from build123d import *

# Parameters (mm, degrees)
SKETCH_1_R          = 1.1
SKETCH_1_W          = 26
SKETCH_1_H          = 32.5
EXTRUDE_1_DEPTH     = 11
SKETCH_3_R          = 1.1
EXTRUDE_2_DEPTH     = 2
SKETCH_2_R          = 1.1
CUT_EXTRUDE_1_DEPTH = 50.401315772
SKETCH_4_W          = 8
SKETCH_4_H          = 17
CUT_EXTRUDE_3_DEPTH = 10
SKETCH_5_R          = 2.5
CUT_EXTRUDE_4_DEPTH = 0.4
SKETCH_6_W          = 3.5
SKETCH_6_H          = 13
SKETCH_6_W_2        = 10
SKETCH_6_H_2        = 2
CUT_EXTRUDE_6_DEPTH = 3
FILLET_1_R          = 7.5
SKETCH_7_W          = 3
SKETCH_7_H          = 13
CUT_EXTRUDE_7_DEPTH = 49.449355001


with BuildPart() as part:
    # ｽｹｯﾁ1 → ﾎﾞｽ - 押し出し1 (new body)
    with BuildSketch(Plane.XY):
        with BuildLine():
            Line((26.8, 35.5), (26.8, -3.5))
            ThreePointArc((26.8, -3.5), (26.067766953, -5.267766953), (24.3, -6))
            Line((24.3, -6), (-2.5, -6))
            ThreePointArc((-2.5, -6), (-4.267766953, -5.267766953), (-5, -3.5))
            Line((-5, -3.5), (-5, 33))
            ThreePointArc((-5, 33), (-4.267766953, 34.767766953), (-2.5, 35.5))
            Line((-2.5, 35.5), (26.8, 35.5))
        make_face()
        with Locations((-2.5, 33)):
            Circle(SKETCH_1_R, mode=Mode.SUBTRACT)
        with Locations((-2.5, -3.5)):
            Circle(SKETCH_1_R, mode=Mode.SUBTRACT)
        with Locations((21.8, -3.5)):
            Circle(SKETCH_1_R, mode=Mode.SUBTRACT)
        with Locations((13, 16.25)):
            Rectangle(SKETCH_1_W, SKETCH_1_H, mode=Mode.SUBTRACT)
    extrude(amount=EXTRUDE_1_DEPTH)

    # ｽｹｯﾁ3 → ﾎﾞｽ - 押し出し2 (add)
    with BuildSketch(Plane(origin=(0, 0, 11), x_dir=(-1, 0, 0), z_dir=(0, 0, -1))):
        with BuildLine():
            Line((5, -3.5), (5, 33))
            ThreePointArc((5, 33), (4.267766953, 34.767766953), (2.5, 35.5))
            Line((2.5, 35.5), (-26.8, 35.5))
            Line((-26.8, 35.5), (-26.8, -3.5))
            ThreePointArc((-26.8, -3.5), (-26.067766953, -5.267766953), (-24.3, -6))
            Line((-24.3, -6), (2.5, -6))
            ThreePointArc((2.5, -6), (4.267766953, -5.267766953), (5, -3.5))
        make_face()
        with Locations((-21.8, -3.5)):
            Circle(SKETCH_3_R, mode=Mode.SUBTRACT)
        with Locations((2.5, -3.5)):
            Circle(SKETCH_3_R, mode=Mode.SUBTRACT)
        with Locations((2.5, 33)):
            Circle(SKETCH_3_R, mode=Mode.SUBTRACT)
    extrude(amount=-EXTRUDE_2_DEPTH)

    # ｽｹｯﾁ2 → ｶｯﾄ - 押し出し1 (cut, through all)
    with BuildSketch(Plane.ZY.offset(5)):
        with Locations(Location((8.5, 30, 0), (0, 0, 270))):
            Circle(SKETCH_2_R)
        with Locations(Location((8.5, 9, 0), (0, 0, 270))):
            Circle(SKETCH_2_R)
    extrude(amount=-CUT_EXTRUDE_1_DEPTH, mode=Mode.SUBTRACT)

    # ｽｹｯﾁ4 → ｶｯﾄ - 押し出し3 (cut)
    with BuildSketch(Plane.XY.offset(13)):
        with Locations((6.5, 18.75)):
            Rectangle(SKETCH_4_W, SKETCH_4_H)
    extrude(amount=-CUT_EXTRUDE_3_DEPTH, mode=Mode.SUBTRACT)

    # ｽｹｯﾁ5 → ｶｯﾄ - 押し出し4 (cut)
    with BuildSketch(Plane(origin=(26.8, 0, 0), x_dir=(0, 0, -1), z_dir=(1, 0, 0))):
        with Locations((-8.5, 30)):
            Circle(SKETCH_5_R)
        with Locations((-8.5, 9)):
            Circle(SKETCH_5_R)
    extrude(amount=-CUT_EXTRUDE_4_DEPTH, mode=Mode.SUBTRACT)

    # ｽｹｯﾁ6 → ｶｯﾄ - 押し出し6 (cut)
    with BuildSketch(Plane(origin=(0, 0, 0), x_dir=(-1, 0, 0), z_dir=(0, 0, -1))):
        with Locations((1.75, 9)):
            Rectangle(SKETCH_6_W, SKETCH_6_H)
        with Locations((-21.8, 34.5)):
            Rectangle(SKETCH_6_W_2, SKETCH_6_H_2)
    extrude(amount=-CUT_EXTRUDE_6_DEPTH, mode=Mode.SUBTRACT)

    # ﾌｨﾚｯﾄ1
    # the kernel refuses this fillet: 7.5 mm, written as the material it adds along each edge
    with BuildSketch(Plane(origin=(16.8, 33.5, 0), x_dir=(0, 1, 0), z_dir=(0, 0, 1))) as fillet_1_piece_1:
        with BuildLine():
            CenterArc((7.5, -5.099019514), FILLET_1_R, 137.166571934, 42.833428066)
            Line((0, -5.099019514), (0, 0))
            Line((0, 0), (2, 0))
        make_face()
    extrude(amount=3)

    # ｽｹｯﾁ7 → ｶｯﾄ - 押し出し7 (cut, through all)
    with BuildSketch(Plane(origin=(-3.5, 0, 0), x_dir=(0, 0, -1), z_dir=(1, 0, 0))):
        with Locations((-1.5, 9)):
            Rectangle(SKETCH_7_W, SKETCH_7_H)
    extrude(amount=CUT_EXTRUDE_7_DEPTH, mode=Mode.SUBTRACT)


solid = part.part
Here's how the part is built. I have some questions about the finished solid (model axes, mm). A direction names the side the tool comes from. Round coordinates to 2 decimals unless told otherwise and drop trailing zeros. Write each loop counter-clockwise with the first axis right and the second up, starting at its lowest first coordinate (ties: lowest second). Pieces come first, ordered by that corner, then holes.
1. Suppose I cut it at D-D (x = 16). List the corners of the cut face in (y, z) for me, and give its area (3 significant figures).
2. Will these pins go through, and if not, where does the flat tip stop? pin 1 Ø5 at (x, y) = (-0.5, 10.5) entering from -Z; pin 2 Ø2.5 at (x, z) = (24, 1.5) entering from +Y; pin 3 Ø1.5 at (y, z) = (7, 1.5) entering from +X.
3. For faces 4 (the cylindrical face through (26.197, 28.984, 8.079)), 5 (the flat face through (2.5, 19, 12)), 6 (the flat face through (-2, 9, 3)), 7 (the flat face through (13, 32.5, 5)), 8 (the cylindrical face through (26.6, 32.11, 7.16)), which set-ups out of +Z, -Z, +X, -X, +Y, -Y let a thin tool reach every point of the face, with its end or its side?
4. Suppose I cut it at B-B (z = 11.75). List the corners of the cut face in (x, y) for me.
5. I need wall thicknesses on L1, parallel to X at y = -3.5, z = 12.25; L2, parallel to Y at x = -2.5, z = 11.95; L3, parallel to X at y = 1, z = 7.5. Which ranges of each line are inside material? Lowest first, please.
6. If we mould it in two halves opening along X, with no side actions, what happens to faces 1 (the flat face through (-3.5, 9, 1)), 2 (the flat face through (-1, 19, 0)), 3 (the flat face through (13, 16, 11))? For each: released by +X, released by -X, zero draft, split by the parting line, or undercut.
7. Suppose I cut it at C-C (y = 9). List the corners of the cut face in (x, z) for me, and give its area (3 significant figures).
8. Suppose I cut it at A-A (y = 17). List the corners of the cut face in (x, z) for me.
Answer sheet:
1. outline: (-6, 0) - (0, 0) - (0, 11) - (32.5, 11) - (32.5, 0) - (35.5, 0) - (35.5, 13) - (-6, 13) - close
1. area: 182 mm2
2. pin 1: stops at z = 3
2. pin 2: stops at y = 33.5
2. pin 3: stops at x = -3.5
3. face 4: +X, -X
3. face 5: +Z, -Z
3. face 6: -Z, +X
3. face 7: -Z
3. face 8: +X
4. outline: (-5, -3.5) arc R2.5 ccw to (-2.5, -6) - (24.3, -6) arc R2.5 ccw to (26.8, -3.5) - (26.8, 35.5) - (-2.5, 35.5) arc R2.5 ccw to (-5, 33) - close; hole circle Ø2.2 at (-2.5, -3.5); hole circle Ø2.2 at (-2.5, 33); hole (2.5, 10.25) - (10.5, 10.25) - (10.5, 27.25) - (2.5, 27.25) - close; hole circle Ø2.2 at (21.8, -3.5)
5. L1: x = -5 to -3.6, -1.4 to 20.7, 22.9 to 26.8
5. L2: y = -6 to -4.6, -2.4 to 31.9, 34.1 to 35.5
5. L3: x = -5 to 0, 26 to 26.8
6. face 1: released by +X
6. face 2: zero draft
6. face 3: undercut
7. outline: (-5, 0) - (-3.5, 0) - (-3.5, 3) - (0, 3) - (0, 7.4) - (-5, 7.4) - close; (-5, 9.6) - (0, 9.6) - (0, 11) - (26, 11) - (26, 9.6) - (26.4, 9.6) - (26.4, 11) - (26.8, 11) - (26.8, 13) - (-5, 13) - close; (26, 3) - (26.8, 3) - (26.8, 6) - (26.4, 6) - (26.4, 7.4) - (26, 7.4) - close
7. area: 101 mm2
8. outline: (-5, 0) - (0, 0) - (0, 11) - (2.5, 11) - (2.5, 13) - (-5, 13) - close; (10.5, 11) - (26, 11) - (26, 0) - (26.8, 0) - (26.8, 13) - (10.5, 13) - close
